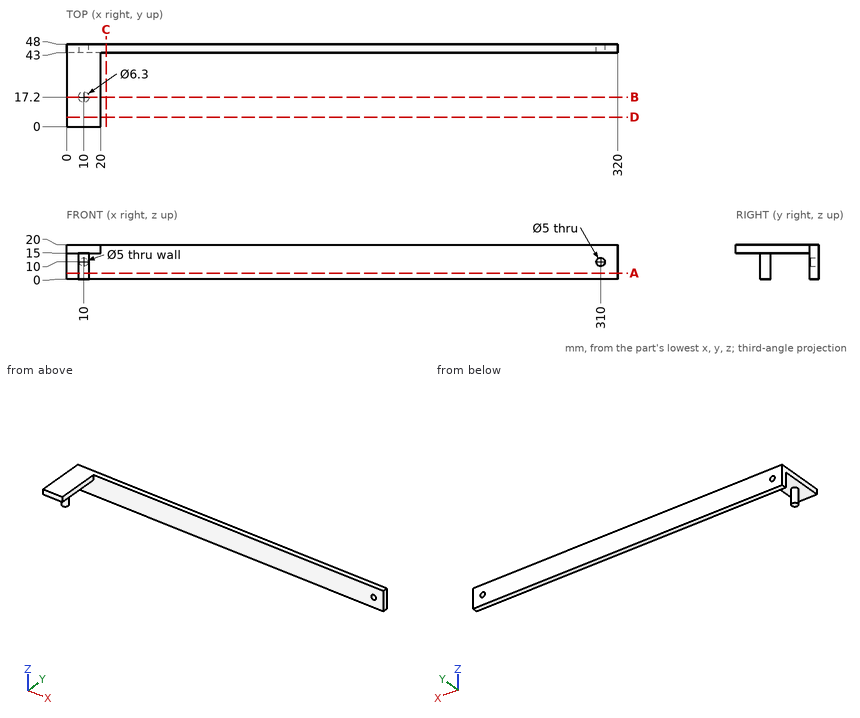
Answer from the drawing. Dimensions are ordinates in mm from the lowest x, y and z of the part. Round coordinates to 2 decimals unless told otherwise and drop trailing zeros. Write each loop counter-clockwise with the first axis right and the second up, starting at its lowest first coordinate (ties: lowest second). Pieces come first, ordered by that corner, then holes. Notation, with made-up numbers: M -22.5,-5 L 11.5,-5 A11 ccw 11.5,14 Z; hole C 72.25,68 d5. An arc over 180 degrees is marked long. One line per item, written item: value.
Q1. Straight lines are drawn through the part: line 1 (X direction, y = 45.55, z = 10); line 2 (Z direction, x = 10, y = 47); line 3 (Y direction, x = 244, z = 5.5). For each, find the intervals that lie inside material, in ascending order. Write a range as [from, to].
Data:
line 1: [0, 7.5], [12.5, 307.5], [312.5, 320]
line 2: [0, 7.5], [12.5, 20]
line 3: [43, 48]
Q2. Find section C-C on x = 23. Write down the section's boundary in (y, z), plus the area to 3 significant figures.
Data:
outline: M 43,0 L 48,0 L 48,20 L 43,20 Z
area: 100 mm2
Q3. Flat-ended cylindrical pins translate along their axes: pin 1 Ø1.5 at (x, z) = (193.5, 6.5) entering from -Y; pin 2 Ø6 at (x, z) = (310, 10) entering from +Y; pin 3 Ø10 at (x, y) = (14, 27) entering from -Z; pin 4 Ø1.5 at (y, z) = (25, 17) entering from +X. Find the tip coordinate at first contact, or state that the pin passes through.
Data:
pin 1: y = 43
pin 2: y = 48
pin 3: z = 15
pin 4: x = 20
Q4. Find section A-A on z = 3.5. Write down the section's boundary in (x, y).
Data:
outline: M 0,43 L 320,43 L 320,48 L 0,48 Z; C 10,17.2 d6.3
Q5. Find section B-B on y = 17.2. Write down the section's boundary in (x, z).
Data:
outline: M 0,15 L 6.85,15 L 6.85,0 L 13.15,0 L 13.15,15 L 20,15 L 20,20 L 0,20 Z
Q6. Find section D-D on y = 5.5. Write down the section's boundary in (x, z), plus the area to 3 significant figures.
Data:
outline: M 0,15 L 20,15 L 20,20 L 0,20 Z
area: 100 mm2
